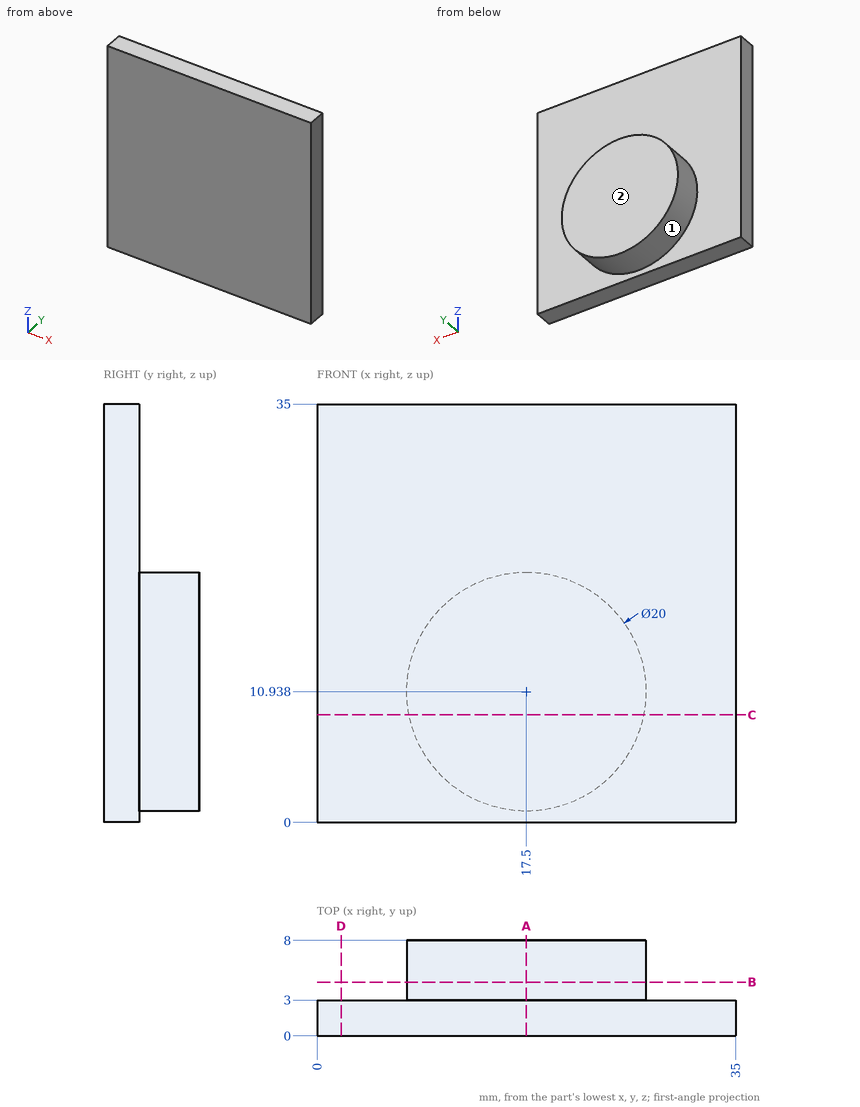
Geometry: see drawing. Coordinates: mm, zero at the bounding-box minimum. A direction names the side the tool comes from. Coordinates: 2 decimals unless noted, no trailing zeros. Loops run counter-clockwise (first coordinate to the right, second up) from the corner with the lowest first, then second, coordinate; pieces in that order, holes last. Notation, with made-up numbers: M 58.5,15.5 L 111.5,15.5 A28 ccw 111.5,36.5 Z; hole C 63,-38 d1. An arc over 180 degrees is marked long. Put each result on its own line as item: value. Start each with the question number.
1) Cut plane C-C on z = 9. Return the cut outline in (x, y).
2) Ray query, L1, parallel to Y at x = 31, z = 14.5; L2, parallel to X at y = 3.5, z = 6 (1 decimal); L3, parallel to Z at x = 23, y = 6 (1 decimal). Return the intervals inside material, ascending. Write a range as from..to.
3) Cut plane D-D on x = 2. Return the cut outline in (y, z).
4) Cut plane B-B on y = 4.5. Return the cut outline in (x, z).
5) Reachability of the marked faces 1 and 2 from +Z, -Z, +X, -X, +Y, -Y: full face, straight path, thin tool, end or side. Return the list, or none.
6) Cut plane A-A on x = 17.5. Return the cut outline in (y, z), then the cut area to 3 significant figures.
The answers:
1. outline: M 0,0 L 35,0 L 35,3 L 27.31,3 L 27.31,8 L 7.69,8 L 7.69,3 L 0,3 Z
2. L1: y = 0..3
2. L2: x = 8.8..26.2
2. L3: z = 2.6..19.3
3. outline: M 0,0 L 3,0 L 3,35 L 0,35 Z
4. outline: C 17.5,10.94 d20
5. face 1: +Y
5. face 2: +Z, -Z, +X, -X, +Y
6. outline: M 0,0 L 3,0 L 3,0.94 L 8,0.94 L 8,20.94 L 3,20.94 L 3,35 L 0,35 Z
6. area: 205 mm²
